```python
from build123d import *

# Parameters (mm, degrees)
SKETCH1_W           = 220
SKETCH1_H           = 150
BOSS_EXTRUDE2_DEPTH = 20
SKETCH3_R           = 10
SKETCH3_R_2         = 9
BOSS_EXTRUDE3_DEPTH = 150
SKETCH4_R           = 9
CUT_EXTRUDE1_DEPTH  = 150


with BuildPart() as part:
    # Sketch1 → Boss-Extrude2 (new body)
    with BuildSketch(Plane(origin=(0, 0, 0), x_dir=(0, 0, -1), z_dir=(1, 0, 0))):
        Rectangle(SKETCH1_W, SKETCH1_H)
    extrude(amount=BOSS_EXTRUDE2_DEPTH)

    # Sketch3 → Boss-Extrude3 (add)
    with BuildSketch(Plane(origin=(0, 75, 0), x_dir=(1, 0, 0), z_dir=(0, 1, 0))):
        with Locations((10, 110)):
            Circle(SKETCH3_R)
        with Locations((10, 110)):
            Circle(SKETCH3_R_2, mode=Mode.SUBTRACT)
    extrude(amount=-BOSS_EXTRUDE3_DEPTH)

    # Sketch4 → Cut-Extrude1 (cut)
    with BuildSketch(Plane(origin=(0, 75, 0), x_dir=(1, 0, 0), z_dir=(0, 1, 0))):
        with Locations(Location((10, 110, 0), (0, 0, 270))):
            Circle(SKETCH4_R)
    extrude(amount=-CUT_EXTRUDE1_DEPTH, mode=Mode.SUBTRACT)


solid = part.part
```
Source: CAD feature listing. Evaluate the final solid. Frame: model axes, mm. Round coordinates to 2 decimals unless told otherwise and drop trailing zeros. Write each loop counter-clockwise with the first axis right and the second up, starting at its lowest first coordinate (ties: lowest second). Pieces come first, ordered by that corner, then holes. Notation, with made-up numbers: M -7,-37 L 37,-37 A29 ccw 37,-17 Z; hole C 19,-1 d1. An arc over 180 degrees is marked long. Use CSV: the item, a comma, the result in double quotes. Start each with the question number.
Q1. First-contact query: P1, Ø6, axis at y = 54.5, z = 73.5, coming from the -X side. Flat tip, straight axial feed; report the tip coordinate or a pass-through.
Q2. Cut plane A-A on x = 10. Output: boundary loops of the cut face in (y, z), plus the area to 3 significant figures.
Q3. Cut plane B-B on y = -24. Output: boundary loops of the cut face in (x, z).
Q4. Line query: line 1 (X direction, y = 17, z = -110); line 2 (Z direction, x = 11, y = 67.5); line 3 (Z direction, x = 3.5, y = 1.5). Output: solid intervals per line, ascending. Write a range as from..to.
Q5. Cut plane C-C on z = -106. Output: boundary loops of the cut face in (x, y), plus the area to 3 significant figures.
Q6. Pull-direction query (Z, two-part tool) for faces 1 (the face through (12.703, 1.05, -101.416)), 2 (the face through (10, -1, 110)), 3 (the face through (20, 1, 2)); classes: +Z half, -Z half, draft (parallel to the pull), parting line (faces both ways), or undercut.
Results found:
1,P1,"x = 0"
2,outline,"M -75,-120 L 75,-120 L 75,-119 L -75,-119 Z; M -75,-101 L 75,-101 L 75,110 L -75,110 Z"
2,area,"31,800 mm^2"
3,outline,"M 0,-110 A10 ccw 20,-110 L 20,110 L 0,110 Z; hole C 10,-110 d18"
4,line 1,"0..1, 19..20"
4,line 2,"-119.95..-118.94, -101.06..110"
4,line 3,"-117.6..-116.22, -103.78..110"
5,outline,"M 0,-75 L 1.94,-75 L 1.94,75 L 0,75 Z; M 18.06,-75 L 20,-75 L 20,75 L 18.06,75 Z"
5,area,"581 mm^2"
6,face 1,"undercut"
6,face 2,"+Z half"
6,face 3,"draft"
